Check sheet for the drawn part. Datum: minimum x, y, z corner. Units: mm. A direction names the side the tool comes from. Coordinates: 2 decimals unless noted, no trailing zeros. Write each loop counter-clockwise with the first axis right and the second up, starting at its lowest first coordinate (ties: lowest second). Pieces come first, ordered by that corner, then holes. Notation, with made-up numbers: (-3.75, 50) -> (16.25, 50) arc R18 cw to (16.25, 55) -> close; hole circle Ø9 at (-14, 82.25). An arc over 180 degrees is marked (long way). One line per question, with ' | ' between items.
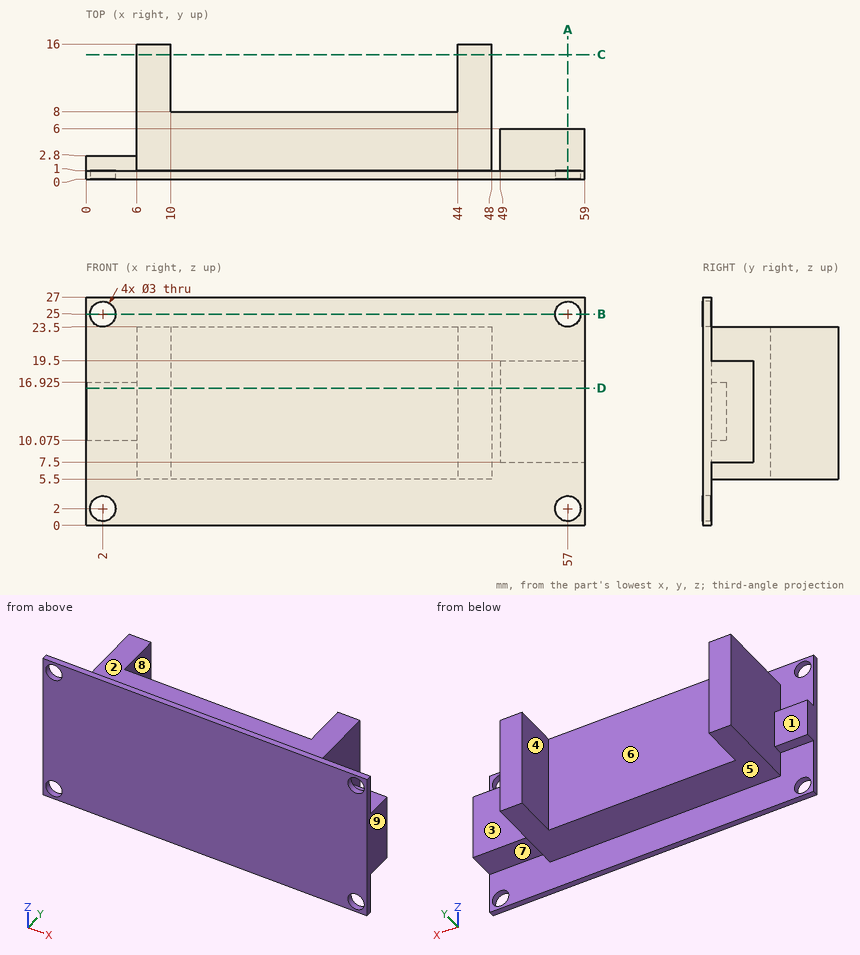
1. Material ranges on line 1 (Z direction, x = 57, y = 0.8); line 2 (X direction, y = 0.8, z = 2); line 3 (X direction, y = 9.75, z = 21.5), recorded low to high. Write a range as from..to.
Worked answers:
line 1: 0..0.5, 3.5..23.5, 26.5..27 | line 2: 0..0.5, 3.5..55.5, 58.5..59 | line 3: 6..10, 44..48
2. Cross-section at D-D on z = 16.25. Record the boundary of the cut face in (x, y), and give its area (3 significant figures).
Worked answers:
outline: (0, 0) -> (59, 0) -> (59, 6) -> (49, 6) -> (49, 1) -> (48, 1) -> (48, 16) -> (44, 16) -> (44, 8) -> (10, 8) -> (10, 16) -> (6, 16) -> (6, 2.8) -> (0, 2.8) -> close | area: 478 mm²
3. Cross-section at A-A on x = 57. Record the boundary of the cut face in (y, z).
Worked answers:
outline: (0, 0) -> (1, 0) -> (1, 0.5) -> (0, 0.5) -> close; (0, 3.5) -> (1, 3.5) -> (1, 7.5) -> (6, 7.5) -> (6, 19.5) -> (1, 19.5) -> (1, 23.5) -> (0, 23.5) -> close; (0, 26.5) -> (1, 26.5) -> (1, 27) -> (0, 27) -> close
4. Cross-section at C-C on y = 14.75. Record the boundary of the cut face in (x, z).
Worked answers:
outline: (6, 5.5) -> (10, 5.5) -> (10, 23.5) -> (6, 23.5) -> close; (44, 5.5) -> (48, 5.5) -> (48, 23.5) -> (44, 23.5) -> close
5. Tool access check on the marked faces 1, 2, 3, 4 and 5. Record the directions out of +Z, -Z, +X, -X, +Y, -Y that give a thin tool (end or side, any length) a straight path to the whole face; none if there is none.
Worked answers:
face 1: +Z, -Z, -X, +Y | face 2: +Z, +X, -X, +Y | face 3: +Z, -Z, +X, +Y | face 4: +Z, -Z, +Y | face 5: -Z, +X, -X, +Y
6. Mould release check, pull along X, two halves, no side actions. Record for the marked faces 6, 7, 8 and 9: released by +X, released by -X, zero draft, split by the parting line, or undercut.
Worked answers:
face 6: undercut | face 7: zero draft | face 8: undercut | face 9: released by +X
7. Cross-section at B-B on z = 25. Record the boundary of the cut face in (x, y), and give its area (3 significant figures).
Worked answers:
outline: (0, 0) -> (0.5, 0) -> (0.5, 1) -> (0, 1) -> close; (3.5, 0) -> (55.5, 0) -> (55.5, 1) -> (3.5, 1) -> close; (58.5, 0) -> (59, 0) -> (59, 1) -> (58.5, 1) -> close | area: 53.0 mm²
8. Go/stop test with flat-tipped pins: P1, Ø5, axis at x = 54, z = 12, coming from the +Y side; P2, Ø1.5, axis at x = 22, z = 14, coming from the -Y side; P3, Ø1.5, axis at x = 39.5, y = 8, coming from the +Z side; P4, Ø2.5, axis at x = 57, z = 2, coming from the +Y side. Record where each tip stops, or that it passes through.
Worked answers:
P1: y = 6 | P2: y = 0 | P3: z = 23.5 | P4: through
